Build history of the part. All positions in model axes, mm. Round coordinates to 2 decimals unless told otherwise and drop trailing zeros. Loops run counter-clockwise (first coordinate to the right, second up) from the corner with the lowest first, then second, coordinate; pieces in that order, holes last.
from build123d import *

# Parameters (mm, degrees)
EXTRUDE1_DEPTH = 0.16
SKETCH4_R      = 0.05
EXTRUDE3_DEPTH = 1.32


with BuildPart() as part:
    # Sketch1 → Extrude1 (new body, symmetric)
    with BuildSketch(Plane(origin=(0, 0, 0), x_dir=(-1, 0, 0), z_dir=(0, 0, -1))):
        Polygon((-4.387, 43.998003308), (4.387, 43.998003308), (7.663262056, 93.984102838), (-7.663262056, 93.984102838), align=None)
    extrude(amount=EXTRUDE1_DEPTH, both=True)

    # Sketch4 → Extrude3 (cut, through all)
    with BuildSketch(Plane.XY.offset(0.16)):
        with Locations((-3, 44.198003308)):
            Circle(SKETCH4_R)
        with Locations((0, 44.198003308)):
            Circle(SKETCH4_R)
        with Locations((3, 44.198003308)):
            Circle(SKETCH4_R)
        with Locations((-5.746391555, 93.784102838)):
            Circle(SKETCH4_R)
        with Locations((0, 93.784102838)):
            Circle(SKETCH4_R)
        with Locations((5.746391555, 93.784102838)):
            Circle(SKETCH4_R)
    extrude(amount=-EXTRUDE3_DEPTH, mode=Mode.SUBTRACT)


solid = part.part
(1) Slice it at A-A on z = -0.1. List the corners of the cut face in (x, y), plus the area to 3 significant figures.
Responses:
outline: (-7.66, 93.98) - (-4.39, 44) - (4.39, 44) - (7.66, 93.98) - close; hole circle Ø0.1 at (-5.75, 93.78); hole circle Ø0.1 at (-3, 44.2); hole circle Ø0.1 at (0, 44.2); hole circle Ø0.1 at (0, 93.78); hole circle Ø0.1 at (3, 44.2); hole circle Ø0.1 at (5.75, 93.78)
area: 602 mm2
(2) Slice it at B-B on y = 74.5. List the corners of the cut face in (x, z), plus the area to 3 significant figures.
Responses:
outline: (-6.39, -0.16) - (6.39, -0.16) - (6.39, 0.16) - (-6.39, 0.16) - close
area: 4.09 mm2
(3) Probe line 1 (X direction, y = 65.5, z = -0.1); line 2 (X direction, y = 67, z = -0.05). List the from-to ranges inside material, lowest first.
Responses:
line 1: x = -5.8 to 5.8
line 2: x = -5.89 to 5.89
(4) Slice it at C-C on x = 6.75. List the corners of the cut face in (y, z), plus the area to 3 significant figures.
Responses:
outline: (80.05, -0.16) - (93.98, -0.16) - (93.98, 0.16) - (80.05, 0.16) - close
area: 4.46 mm2
